Check sheet for the modelled part. Datum: model origin and axes. Units: mm. A direction names the side the tool comes from. Give positions to 0.01 mm unless a question says otherwise; leave off trailing zeros. Loops run counter-clockwise (first coordinate to the right, second up) from the corner with the lowest first, then second, coordinate; pieces in that order, holes last. Notation, with made-up numbers: (50.5, -20) - (57.5, -20) arc R28 cw to (57.5, 5) - close; hole circle Ø4 at (75.25, 68). An arc over 180 degrees is marked (long way). Use CSV: the item, a comma, the result in double quotes.
from build123d import *

# Parameters (mm, degrees)
MAIN_W                 = 20
MAIN_H                 = 12.7
BOSS_EXTRUDE1_DEPTH    = 6.35
M6_5_CLEARANCE_HOLE1_D = 7.1
CUT_EXTRUDE1_DEPTH     = 229.693747182
M8_CLEARANCE_HOLE1_D   = 9
FILLET1_R              = 10


with BuildPart() as part:
    # MAIN → Boss-Extrude1 (new, symmetric)
    # profile 1 of 3: a face of its own
    with BuildSketch(Plane.XY):
        Polygon((92.5, 192.7), (-92.5, 192.7), (-92.5, -132.7), (-92.5, -162.7), (92.5, -162.7), (92.5, -132.7), align=None)
        with Locations((-69.8, 23.65)):
            Rectangle(MAIN_W, MAIN_H, mode=Mode.SUBTRACT)
        with Locations((-69.8, 173.65)):
            Rectangle(MAIN_W, MAIN_H, mode=Mode.SUBTRACT)
        with Locations((69.8, 23.65)):
            Rectangle(MAIN_W, MAIN_H, mode=Mode.SUBTRACT)
        with Locations((69.8, 173.65)):
            Rectangle(MAIN_W, MAIN_H, mode=Mode.SUBTRACT)
    # profile 2 of 3: a face of its own
    with BuildSketch(Plane.XY):
        Polygon((-92.5, -162.7), (-92.5, -132.7), (-122.5, -132.7), (-122.5, -192.7), (-92.5, -192.7), align=None)
    # profile 3 of 3: a face of its own
    with BuildSketch(Plane.XY):
        Polygon((122.5, -132.7), (92.5, -132.7), (92.5, -162.7), (92.5, -192.7), (122.5, -192.7), align=None)
    extrude(amount=BOSS_EXTRUDE1_DEPTH, both=True)

    # M6.5 Clearance Hole1 (through all)
    with Locations(Plane.XY.offset(6.35)):
        with Locations((-107.5, -177.7), (107.5, -177.7)):
            Hole(M6_5_CLEARANCE_HOLE1_D / 2)

    # Sketch1 → Cut-Extrude1 (cut, through all)
    with BuildSketch(Plane.XY.offset(6.35)):
        with BuildLine():
            Line((-67.989745962, -7.782202476), (-76.65, -2.782202476))
            Line((-76.65, -2.782202476), (-75, 0.075681357))
            Line((-75, 0.075681357), (-66.339745962, -4.924318643))
            ThreePointArc((-66.339745962, -4.924318643), (0, -22.7), (66.339745962, -4.924318643))
            Line((66.339745962, -4.924318643), (75, 0.075681357))
            Line((75, 0.075681357), (76.65, -2.782202476))
            Line((76.65, -2.782202476), (67.989745962, -7.782202476))
            ThreePointArc((67.989745962, -7.782202476), (0, -26), (-67.989745962, -7.782202476))
        make_face()
    extrude(amount=-CUT_EXTRUDE1_DEPTH, mode=Mode.SUBTRACT)

    # M8 Clearance Hole1 (through all)
    with Locations(Plane.XY.offset(6.35)):
        with Locations((0, 173.65), (0, 23.65)):
            Hole(M8_CLEARANCE_HOLE1_D / 2)

    # Fillet1
    fillet1_edges = [part.edges().sort_by_distance(p)[0] for p in [
        (-92.5, 192.7, 0),
        (92.5, 192.7, 0),
        (92.5, -132.7, 0),
        (122.5, -132.7, 0),
        (92.5, -192.7, 0),
        (92.5, -162.7, 0),
        (-92.5, -162.7, 0),
        (-92.5, -192.7, 0),
        (-122.5, -132.7, 0),
        (-92.5, -132.7, 0),
    ]]
    fillet(fillet1_edges, radius=FILLET1_R)


solid = part.part
1. Sectioned sample at D-D, the plane y = -50.5. Record the boundary of the cut face in (x, z), and give its area (3 significant figures).
Completed:
outline,"(-92.5, -6.35) - (92.5, -6.35) - (92.5, 6.35) - (-92.5, 6.35) - close"
area,"2,350 mm²"
2. Go/stop test with flat-tipped pins: pin 1 Ø5 at (y, z) = (85, 3.5) entering from +X; pin 2 Ø3 at (y, z) = (-140.5, 5) entering from -X; pin 3 Ø4 at (x, z) = (-70.5, 2.5) entering from -Y. Record where each tip stops, or that it passes through.
Completed:
pin 1,"stops at x = 92.5"
pin 2,"stops at x = -122.48"
pin 3,"stops at y = -162.7"
3. Set-up check for faces 1 (the face through (-89.49, -165.55, -0.09)), 2 (the face through (70, 17.3, 0)), 3 (the face through (119.49, -135.55, -0.09)): record each of +Z, -Z, +X, -X, +Y, -Y from which the full face is reachable in a straight line by a thin tool's end or side.
Completed:
face 1,"+Z, -Z, -Y"
face 2,"+Z, -Z"
face 3,"+Z, -Z, +X, +Y"
4. Sectioned sample at C-C, the plane x = 47. Record the boundary of the cut face in (y, z), and give its area (3 significant figures).
Completed:
outline,"(-162.7, -6.35) - (-17.62, -6.35) - (-17.62, 6.35) - (-162.7, 6.35) - close; (-14.1, -6.35) - (192.7, -6.35) - (192.7, 6.35) - (-14.1, 6.35) - close"
area,"4,470 mm²"
5. Scan lines: line 1 along X through (y, z) = (-177.7, -2.5); line 2 along Y through (x, z) = (0, -1.75); line 3 along X through (y, z) = (167.5, 0.75). Record each from-to range of solid material in increasing order.
Completed:
line 1,"x = -122.5 to -111.05, -103.95 to -92.5, 92.5 to 103.95, 111.05 to 122.5"
line 2,"y = -162.7 to -26, -22.7 to 19.15, 28.15 to 169.15, 178.15 to 192.7"
line 3,"x = -92.5 to -79.8, -59.8 to 59.8, 79.8 to 92.5"
6. Sectioned sample at B-B, the plane x = 0. Record the boundary of the cut face in (y, z), and give its area (3 significant figures).
Completed:
outline,"(-162.7, -6.35) - (-26, -6.35) - (-26, 6.35) - (-162.7, 6.35) - close; (-22.7, -6.35) - (19.15, -6.35) - (19.15, 6.35) - (-22.7, 6.35) - close; (28.15, -6.35) - (169.15, -6.35) - (169.15, 6.35) - (28.15, 6.35) - close; (178.15, -6.35) - (192.7, -6.35) - (192.7, 6.35) - (178.15, 6.35) - close"
area,"4,240 mm²"
7. Release check for a two-part mould opening along X. For faces 4 (the face through (-0.973, -22.696, 0.089)), 5 (the face through (-92.5, 32, 0)), 6 (the face through (92.5, 28, 0)), 7 (the face through (1, 192.7, 0)) record: released by +X, released by -X, zero draft, split by the parting line, or undercut.
Completed:
face 4,"undercut"
face 5,"released by -X"
face 6,"released by +X"
face 7,"zero draft"
8. Sectioned sample at A-A, the plane y = 173.65. Record the boundary of the cut face in (x, z), and give its area (3 significant figures).
Completed:
outline,"(-92.5, -6.35) - (-79.8, -6.35) - (-79.8, 6.35) - (-92.5, 6.35) - close; (-59.8, -6.35) - (-4.5, -6.35) - (-4.5, 6.35) - (-59.8, 6.35) - close; (4.5, -6.35) - (59.8, -6.35) - (59.8, 6.35) - (4.5, 6.35) - close; (79.8, -6.35) - (92.5, -6.35) - (92.5, 6.35) - (79.8, 6.35) - close"
area,"1,730 mm²"
